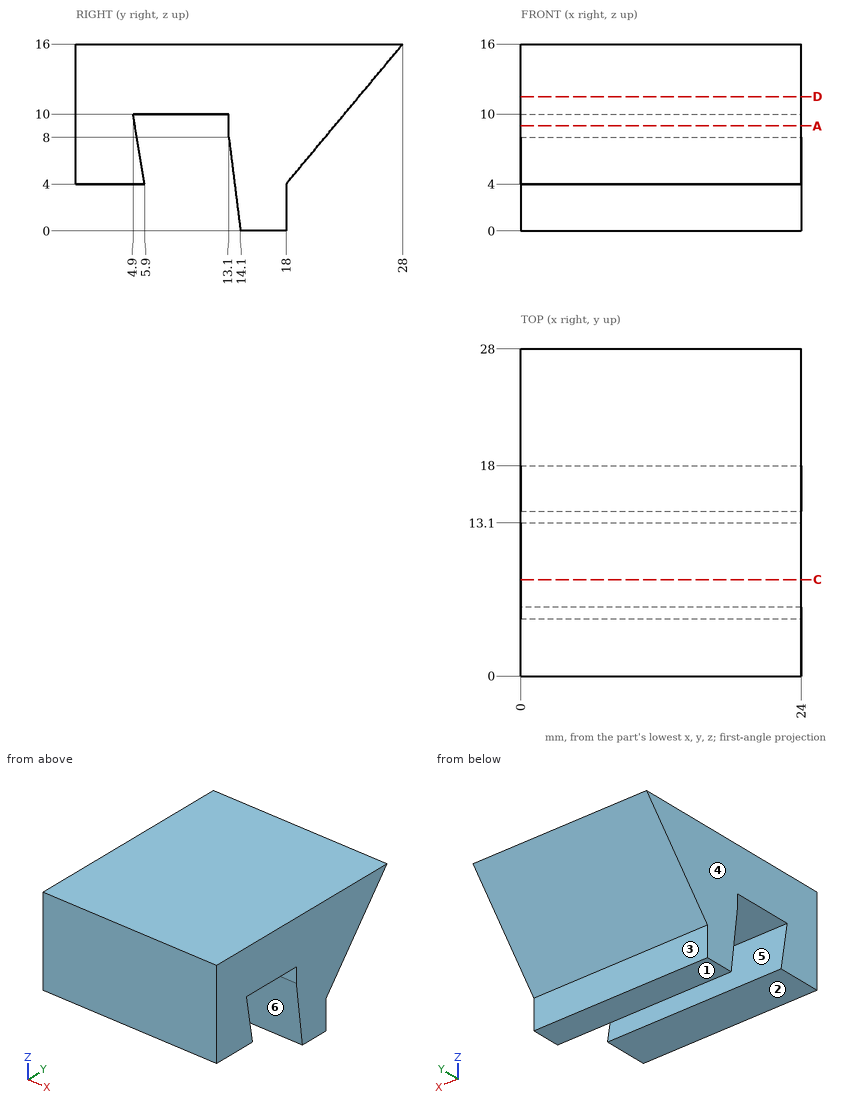
The figure shows three views and two pictorial views of one solid part (mm, origin at its lowest corner). Answer the questions. A direction names the side the tool comes from. Coordinates: 2 decimals unless noted, no trailing zeros. Loops run counter-clockwise (first coordinate to the right, second up) from the corner with the lowest first, then second, coordinate; pieces in that order, holes last. Notation, with made-up numbers: (5, -6.75) - (36, -6.75) arc R12 cw to (36, 12.25) - close; hole circle Ø3 at (77, -4). An arc over 180 degrees is marked (long way). Write item = value, one per line.
1) Section D-D (z = 11.5) is taken. Determine the outline of the cut face in (x, y), plus the area to 3 significant figures.
Responses:
outline = (0, 0) - (24, 0) - (24, 24.25) - (0, 24.25) - close
area = 582 mm^2
2) Find the intervals of material crossed by line 1 along Z through (x, y) = (17.5, 11.75); line 2 along Y through (x, z) = (5, 7) (3 decimals); line 3 along Y through (x, z) = (8, 6), in increasing order.
Responses:
line_1 = 10 to 16
line_2 = 0 to 5.4, 13.225 to 20.5
line_3 = 0 to 5.57, 13.35 to 19.67
3) Which of the six approach directions +Z, -Z, +X, -X, +Y, -Y give full straight-line access (tool end or side, diameter ignored) to the marked faces 1, 2 and 3?
Responses:
face_1 = -Z, +X, -X, +Y, -Y
face_2 = -Z, +X, -X, -Y
face_3 = -Z, +X, -X, +Y
4) Determine the mould class of the marked faces 4, 5 and 6 for opening direction Z: pulls with the +Z half, pulls with the -Z half, needs draft (parallel to the pull), parting line crosses it, or undercut.
Responses:
face_4 = needs draft
face_5 = undercut
face_6 = pulls with the -Z half
5) Section A-A (z = 9) is taken. Determine the outline of the cut face in (x, y).
Responses:
outline = (0, 0) - (24, 0) - (24, 5.07) - (0, 5.07) - close; (0, 13.1) - (24, 13.1) - (24, 22.17) - (0, 22.17) - close
6) Section C-C (y = 8.25) is taken. Determine the outline of the cut face in (x, z), plus the area to 3 significant figures.
Responses:
outline = (0, 10) - (24, 10) - (24, 16) - (0, 16) - close
area = 144 mm^2
7) Each of these flat-tipped pins is pushed along its axis until it touches: P1, Ø6.5, axis at x = 12.5, y = 2.5, coming from the -Z side; P2, Ø2.5, axis at x = 16.5, y = 11, coming from the -Z side; P3, Ø6, axis at x = 19, y = 24.5, coming from the -Z side. Where does it stop, or does it pass through?
Responses:
P1 = 4
P2 = 10
P3 = 8.2
